Autodesk Inventor part; units mm, degrees
ref_plane "YZ Plane" through (0, 0, 0) normal (1, 0, 0) x (0, 1, 0)
ref_plane "XZ Plane" through (0, 0, 0) normal (0, 1, 0) x (-1, 0, 0)
ref_plane "XY Plane" through (0, 0, 0) normal (0, 0, 1) x (1, 0, 0)
sketch "草圖1" plane through (0, 0, 0) normal (0, 0, 1) x (1, 0, 0)
  line L0 (-425, 17.5) -> (425, 17.5)
  line L1 (425, 17.5) -> (425, -17.5)
  line L2 (425, -17.5) -> (-425, -17.5)
  line L3 (-425, -17.5) -> (-425, 17.5)
  point P0 (0, 0)
  dimension "d0" = 850
  dimension "d1" = 35
  dimension "d2" = 17.5
  dimension "d3" = 425
extrude "擠出1" add sketch "草圖1" along normal blind 7.5
sketch "草圖2" plane through (425, -17.5, 0) normal (1, 0, 0) x (0, 0, -1)
  line L0 (0, 35) -> (-7.5, 35)
  line L1 (0, 0) -> (0, 35)
  line L2 (-6, 35) -> (0, 35)
  line L3 (0, 35) -> (0, 32)
  line L4 (0, 32) -> (-6, 32)
  line L5 (-6, 32) -> (-6, 35)
  line L6 (-6, 3) -> (0, 3)
  line L7 (0, 3) -> (0, 0)
  line L8 (0, 0) -> (-6, 0)
  line L9 (-6, 0) -> (-6, 3)
  line L10 (-7.5, 35) -> (-7.5, 0)
  line L11 (-7.5, 30.5) -> (-1, 30.5)
  line L12 (-1, 30.5) -> (-1, 4.5)
  line L13 (-1, 4.5) -> (-7.5, 4.5)
  line L14 (-7.5, 4.5) -> (-7.5, 30.5)
  point P0 (0, 17.5)
  dimension "d6" = 6
  dimension "d7" = 3
  dimension "d8" = 26
  dimension "d9" = 1
  dimension "d10" = 13
extrude "擠出2" cut sketch "草圖2" against normal blind 850
properties part number "鋁軌"
Design review of the part built by this model. Coordinates are the model's own, in mm. Coordinates: 2 decimals unless noted, no trailing zeros. Order: outer loops, then holes, each group sorted by start corner. A loop starts at its lowest first (then second) coordinate and runs counter-clockwise, first axis right, second up. Notation, with made-up numbers: (77, -16) -> (93, -16) arc R25 cw to (93, 5) -> close; hole circle Ø2 at (-15.75, 63). An arc over 180 degrees is marked (long way). One line per item, written item: value. Start each with the question number.
Q1. Mouldability with a two-part tool opening along Y and no side actions: class faces 1 (the flat face through (-6, 0, 0)), 2 (the flat face through (6, 0, 1)) as pulls with the +Y half, pulls with the -Y half, needs draft (parallel to the pull), parting line crosses it, or undercut.
Q2. Take a section at B-B, the plane x = -141. State the section outline as (y, z) points, then the cut area to 3 significant figures.
Q3. Insertion check: pin 1 Ø8 at (x, y) = (0.5, 6) entering from +Z; pin 2 Ø3 at (x, z) = (-139.5, 4) entering from -Y; pin 3 Ø2.5 at (x, y) = (166.5, -16.5) entering from -Z. Each pin has a flat end and moves straight along its axis. Give the tip position at first contact, or say it passes through.
Q4. Take a section at C-C, the plane y = 5.5. State the section outline as (x, z) points.
Q5. For probe 1 along Y at (x, z) = (232, 2); probe 2 along Y at (x, z) = (19.5, 7); probe 3 along Z at (x, y) = (301, -4.5), list the stretches that pass through material, from the lowest coordinate up.
Q6. Take a section at A-A, the plane z = 2.75. State the section outline as (x, y) points, then the cut area to 3 significant figures.
Values follow:
1. face 1: needs draft
1. face 2: undercut
2. outline: (-17.5, 6) -> (-14.5, 6) -> (-14.5, 0) -> (14.5, 0) -> (14.5, 6) -> (17.5, 6) -> (17.5, 7.5) -> (13, 7.5) -> (13, 1) -> (-13, 1) -> (-13, 7.5) -> (-17.5, 7.5) -> close
2. area: 57.5 mm2
3. pin 1: stops at z = 1
3. pin 2: stops at y = -14.5
3. pin 3: stops at z = 6
4. outline: (-425, 0) -> (425, 0) -> (425, 1) -> (-425, 1) -> close
5. probe 1: y = -14.5 to -13, 13 to 14.5
5. probe 2: y = -17.5 to -13, 13 to 17.5
5. probe 3: z = 0 to 1
6. outline: (-425, -14.5) -> (425, -14.5) -> (425, -13) -> (-425, -13) -> close; (-425, 13) -> (425, 13) -> (425, 14.5) -> (-425, 14.5) -> close
6. area: 2,550 mm2
